CAD build for the part. Positions are in the model's coordinates, mm. Face numbers are marked on the shaded views. A direction names the side the tool comes from. Give positions to 0.01 mm unless a question says otherwise; leave off trailing zeros. Order: outer loops, then holes, each group sorted by start corner. A loop starts at its lowest first (then second) coordinate and runs counter-clockwise, first axis right, second up. Notation, with made-up numbers: (-16, 89) -> (34, 89) arc R25 ccw to (34, 125) -> close; hole circle Ø4 at (55, -36). An arc over 180 degrees is marked (long way). Use one line per item in the form item = value. Start each with the question number.
1) Probe line 1 (Y direction, x = 0, z = 1.6); line 2 (Y direction, x = 0, z = 6.1); line 3 (Y direction, x = 24, z = 0.75). List the from-to ranges inside material, lowest first.
2) Cut at A-A, the plane z = 7. Give the cut face in (x, y) (3 decimals).
3) Tool access for the marked faces 1 and 2: list every direction of +Z, -Z, +X, -X, +Y, -Y with a clear straight run to the whole face (end or side of a thin tool).
4) Mould opens along X. For the marked faces 3 and 4 say: pulls with the +X half, pulls with the -X half, needs draft (parallel to the pull), parting line crosses it, or undercut.
5) Drop flat-ended pins along their axis: P1, Ø1.1, axis at x = 35, z = 4.5, coming from the +Y side; P2, Ø1, axis at x = 3.5, z = 4.5, coming from the -Y side. Give the stop position or say it passes through.
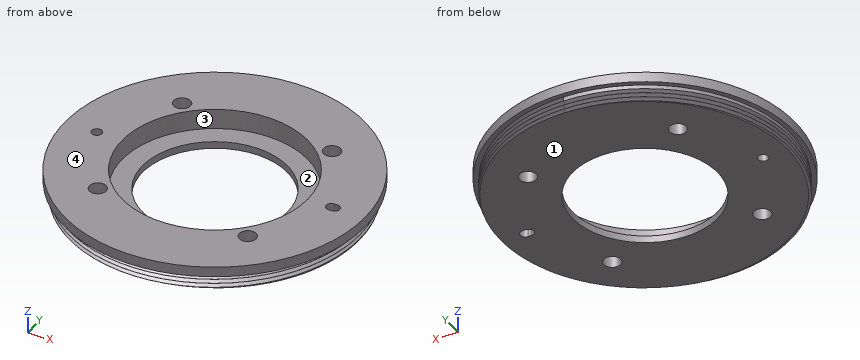
from build123d import *
from build123d.topology import SkipClean

# Parameters (mm, degrees)
SKETCH1_R          = 43
EXTRUDE1_DEPTH     = 5.08
SKETCH2_R          = 44.45
EXTRUDE2_DEPTH     = 3
SKETCH5_R          = 2.5
EXTRUDE4_DEPTH     = 64.378950764
CUT_SWEEP1_PITCH   = 1.27
SKETCH15_R         = 1.51
EXTRUDE10_DEPTH    = 9.525
SKETCH16_R         = 27.5
CUT_EXTRUDE1_DEPTH = 6
SKETCH17_R         = 21.5
CUT_EXTRUDE2_DEPTH = 2.08


with BuildPart() as part:
    # Sketch1 → Extrude1 (new body)
    with BuildSketch(Plane.XY):
        Circle(SKETCH1_R)
    extrude(amount=EXTRUDE1_DEPTH)

    # Sketch2 → Extrude2 (add)
    with BuildSketch(Plane.XY.offset(5.08)):
        Circle(SKETCH2_R)
    extrude(amount=EXTRUDE2_DEPTH)

    # Sketch5 → Extrude4 (cut, through all)
    with BuildSketch(Plane.XY.offset(8.08)):
        with Locations((-22.225, 22.225)):
            Circle(SKETCH5_R)
        with Locations((22.225, 22.225)):
            Circle(SKETCH5_R)
        with Locations((22.225, -22.225)):
            Circle(SKETCH5_R)
        with Locations((-22.225, -22.225)):
            Circle(SKETCH5_R)
    extrude(amount=-EXTRUDE4_DEPTH, mode=Mode.SUBTRACT)

    # Cut-Sweep1: the profile of Sketch10 profile screwed along a right-hand helix of 4 turns, 8 arcs to a turn; built about Z, then put on its axis
    with SkipClean():  # the faces are left unmerged after this step: merging them gives an invalid solid
        cut_sweep1_z = Axis((0, 0, 0), (0, 0, 1))
        cut_sweep1_corners = [(43.0003, 0, -0.625173205), (41.917468245, 0, 0), (43.0003, 0, 0.625173205)]
        with BuildLine(mode=Mode.PRIVATE) as cut_sweep1_profile:
            Line(cut_sweep1_corners[0], cut_sweep1_corners[1])
            Line(cut_sweep1_corners[1], cut_sweep1_corners[2])
            Line(cut_sweep1_corners[2], cut_sweep1_corners[0])
        cut_sweep1_cap = Face(cut_sweep1_profile.wire())
        cut_sweep1_turn_angles = [0, 22.5, 45, 67.5, 90, 112.5, 135, 157.5, 180, 202.5, 225, 247.5, 270, 292.5, 315, 337.5, 360]
        cut_sweep1_turn_weights = [1, 0.9238795325112867, 1, 0.9238795325112867, 1, 0.9238795325112867, 1, 0.9238795325112867, 1, 0.9238795325112867, 1, 0.9238795325112867, 1, 0.9238795325112867, 1, 0.9238795325112867, 1]
        cut_sweep1_turn_rails = [Edge.make_bspline([Vector(p[0], p[1], 0).rotate(cut_sweep1_z, cut_sweep1_turn_angles[k]) / cut_sweep1_turn_weights[k] + Vector(0, 0, p[2] + CUT_SWEEP1_PITCH * cut_sweep1_turn_angles[k] / 360) for k in range(17)], [0, 0, 0, 1, 1, 2, 2, 3, 3, 4, 4, 5, 5, 6, 6, 7, 7, 8, 8, 8], 2, cut_sweep1_turn_weights) for p in cut_sweep1_corners]
        cut_sweep1_turn_sides = [Face.make_surface_from_curves(cut_sweep1_turn_rails[p[0]], cut_sweep1_turn_rails[p[1]]) for p in [(0, 1), (1, 2), (2, 0)]]
        cut_sweep1 = Plane(origin=(0, 0, 4.455), x_dir=(0, 1, 0), z_dir=(0, 0, -1)) * Solid(Shell([*[p.moved(Location((0, 0, CUT_SWEEP1_PITCH * i))) for i in range(4) for p in cut_sweep1_turn_sides], cut_sweep1_cap, cut_sweep1_cap.rotate(cut_sweep1_z, 1440).moved(Location((0, 0, CUT_SWEEP1_PITCH * 1440 / 360)))]))
        add(cut_sweep1, mode=Mode.SUBTRACT)

    # Sketch15 → Extrude10 (cut)
    with SkipClean():  # the faces are left unmerged after this step: merging them gives an invalid solid
        with BuildSketch(Plane(origin=(0, 0, 0), x_dir=(-1, 0, 0), z_dir=(0, 0, -1))):
            with Locations((35, 0)):
                Circle(SKETCH15_R)
            with BuildLine():
                Line((-35.5, 1.51), (-34.5, 1.51))
                ThreePointArc((-34.5, 1.51), (-32.99, 0), (-34.5, -1.51))
                Line((-34.5, -1.51), (-35.5, -1.51))
                ThreePointArc((-35.5, -1.51), (-37.01, 0), (-35.5, 1.51))
            make_face()
        extrude(amount=-EXTRUDE10_DEPTH, mode=Mode.SUBTRACT)

    # Sketch16 → Cut-Extrude1 (cut)
    with SkipClean():  # the faces are left unmerged after this step: merging them gives an invalid solid
        with BuildSketch(Plane.XY.offset(8.08)):
            Circle(SKETCH16_R)
        extrude(amount=-CUT_EXTRUDE1_DEPTH, mode=Mode.SUBTRACT)

    # Sketch17 → Cut-Extrude2 (cut)
    with SkipClean():  # the faces are left unmerged after this step: merging them gives an invalid solid
        with BuildSketch(Plane.XY.offset(2.08)):
            Circle(SKETCH17_R)
        extrude(amount=-CUT_EXTRUDE2_DEPTH, mode=Mode.SUBTRACT)


solid = part.part
Result:
q1.line_1 = -42.47 to -21.5, 21.5 to 42.46
q1.line_2 = -44.45 to -27.5, 27.5 to 44.45
q1.line_3 = -35.67 to -23.99, -20.46 to 20.46, 23.99 to 34.85
q2.outline = circle Ø88.9 at (0, 0); hole circle Ø3.02 at (-35, 0); hole circle Ø55 at (0, 0); hole circle Ø5 at (-22.225, -22.225); hole circle Ø5 at (-22.225, 22.225); hole circle Ø5 at (22.225, -22.225); hole circle Ø5 at (22.225, 22.225); hole (34.5, -1.51) -> (35.5, -1.51) arc R1.51 ccw to (35.5, 1.51) -> (34.5, 1.51) arc R1.51 ccw to start
q3.face_1 = -Z, +X, -X, +Y, -Y
q3.face_2 = +Z
q4.face_3 = undercut
q4.face_4 = needs draft
q5.P1 = 25.51
q5.P2 = -42.9
